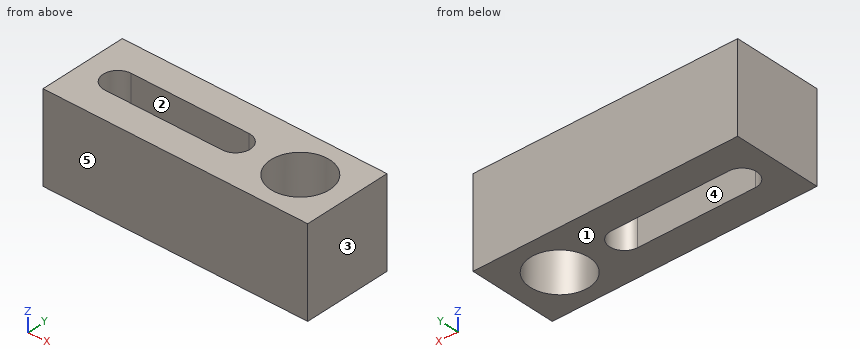
```python
from build123d import *

# Parameters (mm, degrees)
SKETCH1_W           = 45
SKETCH1_H           = 15
SKETCH1_R           = 5
BOSS_EXTRUDE1_DEPTH = 15


with BuildPart() as part:
    # Sketch1 → Boss-Extrude1 (new body)
    with BuildSketch(Plane.XY):
        Rectangle(SKETCH1_W, SKETCH1_H)
        with Locations((14.5, 0)):
            Circle(SKETCH1_R, mode=Mode.SUBTRACT)
        with BuildLine():
            Line((3.5, -2.5), (-16.5, -2.5))
            ThreePointArc((-16.5, -2.5), (-19, 0), (-16.5, 2.5))
            Line((-16.5, 2.5), (3.5, 2.5))
            ThreePointArc((3.5, 2.5), (6, 0), (3.5, -2.5))
        make_face(mode=Mode.SUBTRACT)
    extrude(amount=BOSS_EXTRUDE1_DEPTH)


solid = part.part
```
Verification items for the finished model (mm, model axes). Face numbers are marked on the shaded views. A direction names the side the tool comes from. Give positions to 0.01 mm unless a question says otherwise; leave off trailing zeros. Loops run counter-clockwise (first coordinate to the right, second up) from the corner with the lowest first, then second, coordinate; pieces in that order, holes last.
1. Thickness scan on line 1 (Y direction, x = 14.5, z = 10); line 2 (Y direction, x = -5, z = 13.25); line 3 (X direction, y = 0.5, z = 5.75). Record the ranges inside material, lowest first.
2. Section check B-B, the plane x = -6.5. Enter the section's corners in (y, z).
3. Section check A-A, the plane y = -3. Enter the section's corners in (x, z).
4. Set-up check for the marked faces 1 and 2: record each of +Z, -Z, +X, -X, +Y, -Y from which the full face is reachable in a straight line by a thin tool's end or side.
5. Mould release check, pull along X, two halves, no side actions. Record for the marked faces 3, 4 and 5: released by +X, released by -X, zero draft, split by the parting line, or undercut.
6. Section check C-C, the plane z = 12. Enter the section's corners in (x, y).
7. Section check D-D, the plane y = -1. Enter the section's corners in (x, z).
Geometry says:
1. line 1: y = -7.5 to -5, 5 to 7.5
1. line 2: y = -7.5 to -2.5, 2.5 to 7.5
1. line 3: x = -22.5 to -18.95, 5.95 to 9.53, 19.47 to 22.5
2. outline: (-7.5, 0) - (-2.5, 0) - (-2.5, 15) - (-7.5, 15) - close; (2.5, 0) - (7.5, 0) - (7.5, 15) - (2.5, 15) - close
3. outline: (-22.5, 0) - (10.5, 0) - (10.5, 15) - (-22.5, 15) - close; (18.5, 0) - (22.5, 0) - (22.5, 15) - (18.5, 15) - close
4. face 1: -Z, +X, -X, +Y, -Y
4. face 2: +Z, -Z
5. face 3: released by +X
5. face 4: undercut
5. face 5: zero draft
6. outline: (-22.5, -7.5) - (22.5, -7.5) - (22.5, 7.5) - (-22.5, 7.5) - close; hole (-16.5, -2.5) - (3.5, -2.5) arc R2.5 ccw to (3.5, 2.5) - (-16.5, 2.5) arc R2.5 ccw to start; hole circle Ø10 at (14.5, 0)
7. outline: (-22.5, 0) - (-18.79, 0) - (-18.79, 15) - (-22.5, 15) - close; (5.79, 0) - (9.6, 0) - (9.6, 15) - (5.79, 15) - close; (19.4, 0) - (22.5, 0) - (22.5, 15) - (19.4, 15) - close
